Autodesk Inventor part; units mm, degrees
ref_plane "YZ Plane" through (0, 0, 0) normal (1, 0, 0) x (0, 1, 0)
ref_plane "XZ Plane" through (0, 0, 0) normal (0, 1, 0) x (-1, 0, 0)
ref_plane "XY Plane" through (0, 0, 0) normal (0, 0, 1) x (1, 0, 0)
sketch "Sketch2" plane through (0, 0, 0) normal (0, 1, 0) x (-1, 0, 0)
  line L0 (-5.5536, -11.7431) -> (5.5568, -15.0764)
  line L1 (5.5568, -25.2431) -> (-23.9154, -25.2431)
  line L2 (-23.9154, -25.2431) -> (-23.9154, -11.7431)
  line L3 (-5.5536, -11.7431) -> (-23.9154, -11.7431)
  line L4 (5.5568, -25.2431) -> (5.5568, -15.0764)
  circle A0 centre (-23.9154, -18.4931) radius 6.75
  circle A1 centre (-23.9154, -18.4931) radius 2.2
  circle A2 centre (-23.9154, -18.4931) radius 6.202
  circle A3 centre (-24.9154, -18.9931) radius 6.25
  line L5 (-18.8553, -31.0955) -> (-18.419, -3.4058)
  point P0 (0, 0)
  point P1 (0, 0)
  point P2 (-19.4912, -10.8803)
  point P3 (-19.4912, -24.3803)
  point P4 (-23.9154, -12.2912)
  point P5 (-23.9154, -24.6951)
  dimension "d1" = 13.5
  dimension "d0" = 4.4
  dimension "d6" = 0.5
  dimension "d7" = 1
  dimension "d8" = 12.5
extrude "Extrusion1" add sketch "Sketch2" along normal blind 3.85 contours L0 L4 L1 L5 A0 L3 | L5 A0 L3 | A0 L5 A2 L2 | L2 A2 A3 A0 | A0 L5 A2 | L1 A0 L5 | A2 L5 A3 L2 | L2 A3 A2 | A3 A2 L2 A0 | L5 A2 A3 | A2 L5 | A0 A3 L2 | L2 A3 A2 L5 A0 | A3 A2 L2 A1 | L2 A1 A2 A3 | L2 A2 A3
extrude "Extrusion2" add sketch "Sketch2" along normal blind 8.85 contours L0 L4 L1 L5 A0 L3 | L5 A0 L3 | A0 L5 A2 L2 | A0 L5 A2 | L1 A0 L5 | L2 A3 A2 L5 A0 | L2 A2 A3 picked at (-23.6214, -24.9369)
sketch "Sketch3" plane through (0, 8.85, 0) normal (0, 1, 0) x (1, 0, 0)
  line L0 (-5.5568, 25.2431) -> (-5.5568, 15.0764)
  line L1 (-5.5568, 15.0764) -> (5.5536, 11.7431)
  line L2 (5.5536, 11.7431) -> (23.9154, 11.7431)
  line L3 (23.9154, 11.7431) -> (23.9154, 12.2912)
  arc A0 (23.9154, 24.6951) -> (23.9154, 12.2912) centre (23.9154, 18.4931) ccw
  line L4 (23.9154, 24.6951) -> (23.9154, 25.2431)
  line L5 (23.9154, 25.2431) -> (-5.5568, 25.2431)
  line L6 (18.8553, 31.0955) -> (18.419, 3.4058)
  point P0 (0, 0)
  point P1 (18.6062, 15.2873)
  point P2 (18.5504, 11.7431)
  point P3 (18.7631, 25.2431)
  point P4 (18.7099, 21.8646)
extrude "Extrusion3" cut sketch "Sketch3" against normal up to surface (5 mm away) contours L5 L4 A0 L6 | L6 A0 L3 L2
sketch "Sketch4" plane through (-5.5568, 0, -25.2431) normal (-1, 0, 0) x (0, 0, 1)
  line L0 (0, 0) -> (10.1667, 0)
  line L1 (10.1667, 0) -> (10.1667, 8.85)
  line L2 (0, 8.85) -> (10.1667, 8.85)
  line L3 (0, 0) -> (0, 8.85)
  line L4 (9.1667, 7.85) -> (9.1667, 1)
  line L5 (9.1667, 1) -> (1, 1)
  line L6 (1, 1) -> (1, 7.85)
  line L7 (1, 7.85) -> (9.1667, 7.85)
  point P0 (25.2431, 0)
  dimension "d11" = 1
extrude "Extrusion4" cut sketch "Sketch4" against normal blind 8 contours L4 L5 L6 L7
sketch "Sketch5" plane through (-5.5568, 1, -16.0764) normal (0, 1, 0) x (1, 0, 0)
  line L0 (0, 0) -> (0, 8.1667)
  line L1 (0, 0) -> (8, 0)
  line L2 (8, 0) -> (8, 8.1667)
  line L3 (0, 8.1667) -> (8, 8.1667)
  line L4 (8, 4.0834) -> (2.9855, 4.0834) construction
  line L5 (4, 0) -> (4, 4.0834) construction
  circle A0 centre (4, 4.0834) radius 2.55
  point P0 (5.5568, -16.0764)
  dimension "d14" = 5.1
extrude "Extrusion5" add sketch "Sketch5" along normal up to surface (6.85 mm away) contours A0
sketch "Sketch6" plane through (5.5536, 0, -11.7431) normal (0, 0, 1) x (1, 0, 0)
  line L0 (-11.1104, 7.85) -> (-11.1104, 1)
  line L1 (-11.1104, 7.85) -> (-4.8007, 7.85)
  line L2 (-4.8007, 7.85) -> (-4.8007, 1)
  line L3 (-11.1104, 1) -> (-4.8007, 1)
  point P0 (-5.5536, 0)
extrude "Extrusion6" cut sketch "Sketch6" against normal up to surface (4.3333 mm away)
sketch "Sketch7" plane through (-5.5568, 1, -24.2431) normal (0, 0, 1) x (1, 0, 0)
  line L0 (0, 0) -> (0, 6.85)
  line L1 (0, 0) -> (8, 0)
  line L2 (8, 0) -> (8, 6.85)
  line L3 (0, 6.85) -> (8, 6.85)
  point P0 (5.5568, -1)
extrude "Extrusion7" cut sketch "Sketch7" against normal blind 10.25
sketch "Sketch8" plane through (0, 8.85, 0) normal (0, 1, 0) x (1, 0, 0)
  circle A0 centre (-1.5568, 20.1598) radius 2.55
  circle A1 centre (-1.5568, 20.1598) radius 2.55
  line L0 (-5.5568, 25.2431) -> (2.4432, 25.2431)
  point P0 (0, 0)
fillet "Fillet1" radius 3 2 edges at (-5.5568, 8.35, -15.0764) (-5.5568, 0.5, -15.0764)
chamfer "Chamfer1" distance 2 angle 45 2 edges at (-5.5568, 8.35, -25.2431) (-5.5568, 0.5, -25.2431)
chamfer "Chamfer2" distance 2 angle 45 1 edges at (18.7631, 6.35, -25.2431)
fillet "Fillet2" radius 3 1 edges at (18.5504, 6.35, -11.7431)
sketch "Sketch9" plane through (0, 3.85, 0) normal (0, 1, 0) x (1, 0, 0)
  arc A0 (23.9154, 11.7431) -> (23.9154, 25.2431) centre (23.9154, 18.4931) ccw
  line L0 (16.7631, 25.2431) -> (23.9154, 25.2431)
  line L1 (18.7316, 23.2434) -> (16.7631, 25.2431)
  line L2 (18.7099, 21.8646) -> (18.7316, 23.2434)
  arc A1 (18.7099, 21.8646) -> (18.6062, 15.2873) centre (23.9154, 18.4931) ccw
  line L3 (18.5969, 14.6959) -> (18.6062, 15.2873)
  arc A2 (15.5973, 11.7431) -> (18.5969, 14.6959) centre (15.5973, 14.7431) ccw
  line L4 (23.9154, 11.7431) -> (15.5973, 11.7431)
  circle A3 centre (23.9154, 18.4931) radius 2.2
  point P0 (0, 0)
extrude "Extrusion8" add sketch "Sketch9" against normal blind 3.85 from surface at 5
extrude "Extrusion9" cut sketch "Sketch9" against normal blind 10
chamfer "Chamfer4" distance 1 angle 45 9 edges at (17.7142, 0, -18.5909) (17.7018, 0, -12.6052) (10.5754, 0, -11.7431) (18.6016, 0, -14.9916) (17.7474, 0, -24.2433) (6.6031, 0, -25.2431) (10.1793, 8.85, -25.2431) (30.6654, 8.85, -18.4931) (14.7345, 8.85, -11.7431)
fillet "Fillet3" radius 1 2 edges at (-4.1068, 7.85, -20.1598) (-4.1068, 1, -20.1598)
ref_plane "Work Plane1" through (0, 4.425, 0) normal (0, -1, 0) x (1, 0, 0)
properties part number "Upper Leg_oposite"
Geometry: final body of the model. Coordinates: model frame, mm. A direction names the side the tool comes from. Give positions to 0.01 mm unless a question says otherwise; leave off trailing zeros. Write each loop counter-clockwise with the first axis right and the second up, starting at its lowest first coordinate (ties: lowest second). Pieces come first, ordered by that corner, then holes. Notation, with made-up numbers: M 67,57.5 L 78,57.5 A18 cw 78,84.5 Z; hole C 35,26.5 d4. An arc over 180 degrees is marked long. Answer in a Markdown table with one row per item. Add a question column.
(1) Ray query, line 1 (Y direction, x = -2, z = -14.25); line 2 (Y direction, x = 25.5, z = -22.5); line 3 (X direction, y = 3, z = -21.5). Return the intervals inside material, ascending.
(2) First-contact query: pin 1 (4 mm diameter, centred on x = 23.92, z = -18.49, fed in from -Y); pin 2 (1.5 mm diameter, centred on x = 18.5, z = -17, fed in from -Y); pin 3 (5 mm diameter, centred on y = 4, z = -20.5, fed in from +X); pin 4 (0.8 mm diameter, centred on x = 1.5, y = 4, fed in from -Z). Flat tips, straight axial feed; report the tip coordinate or a pass-through.
(3) Section A-A on y = 5.5. Return loops of the section in (x, z).
(4) Section B-B on x = 7. Return loops of the section in (y, z).
(5) Section C-C on y = 7.25. Return loops of the section in (x, z), and give its area (3 significant figures).
(6) Mould query, pull axis Z, two halves, no side actions, for faces 6 (the cylindrical face through (17.715, 2.445, -18.639)), 7 (the flat face through (2.13, 4.36, -12.77)), 8 (the flat face through (12, 8.85, -19)). Classes: +Z half, -Z half, draft (parallel to the pull), parting line (faces both ways), or undercut.
(7) Section D-D on z = -19.25. State how many separate pieces and enclosed holes the cut face has, and give its area (3 significant figures).
(8) Reachability of faces 1 (the flat face through (-2, 1, -16)), 2 (the flat face through (9.879, 8.357, -24.736)), 3 (the cylindrical face through (17.725, 4.417, -12.628)), 4 (the flat face through (2.443, 4, -21)), 5 (the cylindrical face through (17.714, 4.417, -18.542)) from +Z, -Z, +X, -X, +Y, -Y: full face, straight path, thin tool, end or side. Return the list, or none.
Result set:
| question | item | result |
|---|---|---|
| 1 | line 1 | y = 0 to 1, 7.85 to 8.85 |
| 1 | line 2 | y = 5 to 8.85 |
| 1 | line 3 | x = -3.73 to 0.61, 2.44 to 18.49 |
| 2 | pin 1 | passes through |
| 2 | pin 2 | stops at y = 0.83 |
| 2 | pin 3 | stops at x = 30.67 |
| 2 | pin 4 | stops at z = -16.08 |
| 3 | outline | C -1.56,-20.16 d5.1; M 0.75,-16.08 L 2.44,-16.08 L 2.44,-25.24 L 23.92,-25.24 A6.75 ccw 23.92,-11.74 L 5.55,-11.74 L 0.75,-13.18 Z; hole C 23.92,-18.49 d4.4 |
| 4 | outline | M 0,-24.24 L 1,-25.24 L 7.85,-25.24 L 8.85,-24.24 L 8.85,-12.74 L 7.85,-11.74 L 1,-11.74 L 0,-12.74 Z |
| 5 | outline | C -1.56,-20.16 d5.27; M 0.75,-16.08 L 2.44,-16.08 L 2.44,-25.24 L 23.92,-25.24 A6.75 ccw 23.92,-11.74 L 5.55,-11.74 L 0.75,-13.18 Z; hole C 23.92,-18.49 d4.4 |
| 5 | area | 372 mm^2 |
| 6 | face 6 | undercut |
| 6 | face 7 | +Z half |
| 6 | face 8 | draft |
| 7 | separate pieces | 2 |
| 7 | enclosed holes | 1 |
| 7 | area | 218 mm^2 |
| 8 | face 1 | none |
| 8 | face 2 | -Z, +X, -X, +Y |
| 8 | face 3 | +Z, +X, -Y |
| 8 | face 4 | -Z |
| 8 | face 5 | +X, -Y |
